The figure shows three views and two pictorial views of one solid part (mm, origin at its lowest corner). Answer the questions. Coordinates: 2 decimals unless noted, no trailing zeros. Order: outer loops, then holes, each group sorted by start corner. A loop starts at its lowest first (then second) coordinate and runs counter-clockwise, first axis right, second up. Notation, with made-up numbers: (9.25, 22.25) -> (65.25, 22.25) arc R22 cw to (65.25, 58.25) -> close; hole circle Ø1 at (49.25, -13). An arc over 180 degrees is marked (long way). Return JSON: item names as keys, results as strings.
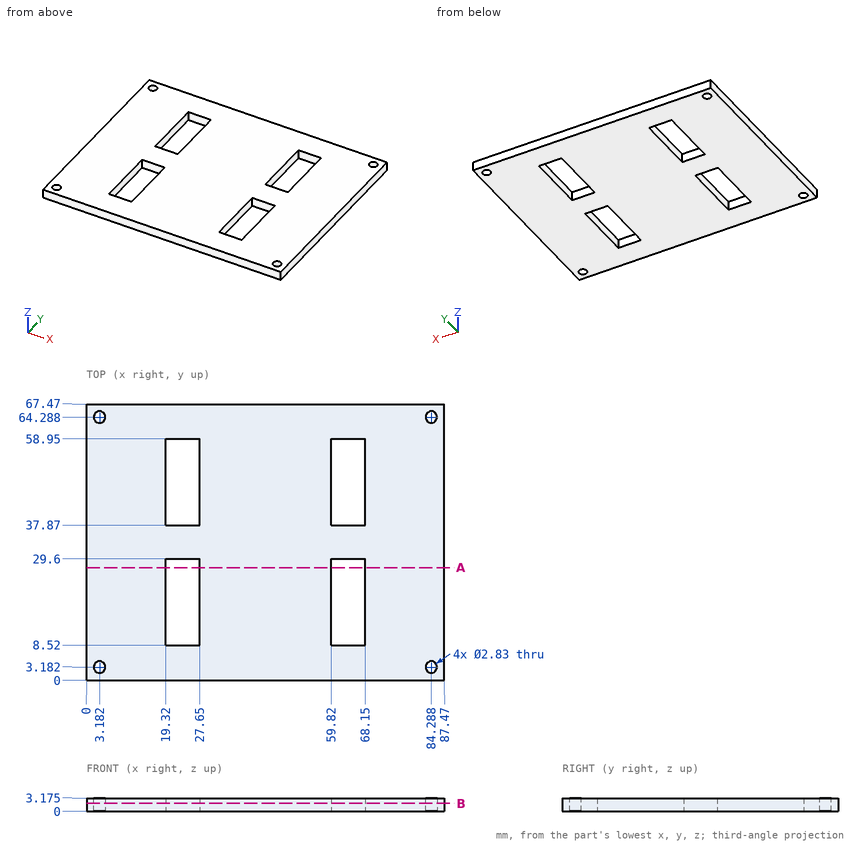
Item 1: Find the intervals of material crossed by probe 1 along X at (y, z) = (50.5, 1.4); probe 2 along X at (y, z) = (3, 2.55); probe 3 along Y at (x, z) = (84, 2.25), in increasing order.
Answer list:
{"probe 1": "0 to 19.32, 27.65 to 59.82, 68.15 to 87.47", "probe 2": "0 to 1.78, 4.59 to 82.88, 85.69 to 87.47", "probe 3": "0 to 1.8, 4.57 to 62.9, 65.67 to 67.47"}
Item 2: The part is cut by section A-A on y = 27.5. Determine the outline of the cut face in (x, z) (3 decimals), plus the area to 3 significant figures.
Answer list:
{"outline": "(0, 0) -> (19.32, 0) -> (19.32, 3.175) -> (0, 3.175) -> close; (27.65, 0) -> (59.82, 0) -> (59.82, 3.175) -> (27.65, 3.175) -> close; (68.15, 0) -> (87.47, 0) -> (87.47, 3.175) -> (68.15, 3.175) -> close", "area": "225 mm2"}
Item 3: The part is cut by section B-B on z = 1.9. Count the separate pieces of the cut face and the enclosed holes in it, plus the area to 3 significant figures.
Answer list:
{"separate pieces": "1", "enclosed holes": "8", "area": "5,170 mm2"}
